Here's how the part is built. I have some questions about the finished solid (model axes, mm). A direction names the side the tool comes from. Coordinates: 2 decimals unless noted, no trailing zeros. Write each loop counter-clockwise with the first axis right and the second up, starting at its lowest first coordinate (ties: lowest second). Pieces come first, ordered by that corner, then holes.
Item 1: Please list where these lines run through material, in increasing order: line 1 (X direction, y = 0.5, z = 3); line 2 (Z direction, x = 6.25, y = -1.5); line 3 (X direction, y = 2, z = -0.75).
Item 2: I'm going to push flat-ended pins straight in: P1, Ø1, axis at y = 2.5, z = 1.5, coming from the +X side; P2, Ø1, axis at x = 2.5, y = -1, coming from the +Z side; P3, Ø1.5, axis at x = 3.5, y = 2, coming from the +Z side. Where does each tip first touch, or does it pass through?
Item 3: I want a section at C-C (x = 5.75). Please give me the cut outline in (y, z).
Item 4: I want a section at A-A (z = 0). Please give me the cut outline in (x, y).
Item 5: If we mould it in two halves opening along X, with no side actions, what happens to faces 1 (the face through (4, 2, 0)), 2 (the face through (7, 0, 0)), 3 (the face through (1, 2, 2)), 4 (the face through (6.3, -0.1, -2.5))? For each: pulls with the +X half, pulls with the -X half, needs draft (parallel to the pull), parting line crosses it, or undercut.
Item 6: For faces 5 (the face through (6, -2, 1)), 6 (the face through (0, 0, 0)), which set-ups out of +Z, -Z, +X, -X, +Y, -Y let a thin tool reach every point of the face, with its end or its side?
from build123d import *

# Parameters (mm, degrees)
SMUSSO1_SIZE = 0.5


with BuildPart() as part:
    # Schizzo1 → Rivoluzione1 (revolve)
    with BuildSketch(Plane.XY, mode=Mode.PRIVATE) as rivoluzione1_sk:
        Polygon((0, 0), (0, 3.75), (1, 3.75), (1, 2), (6, 2), (6, 2.5), (7, 2.5), (7, 0), align=None)
    revolve(rivoluzione1_sk.sketch.rotate(Axis((-5.173483989, 0, 0), (1, 0, 0)), 90), axis=Axis((-5.173483989, 0, 0), (1, 0, 0)))

    # Smusso1
    smusso1_edges = [part.edges().sort_by_distance(p)[0] for p in [
        (7, 0, -2.5),
        (0, 0, -3.75),
    ]]
    chamfer(smusso1_edges, length=SMUSSO1_SIZE)


solid = part.part
Answer:
1. line 1: x = 0 to 1
1. line 2: z = -2 to 2
1. line 3: x = 0 to 1, 6 to 6.86
2. P1: stops at x = 6.58
2. P2: stops at z = 1.94
2. P3: stops at z = 1.56
3. outline: circle Ø4 at (0, 0)
4. outline: (0, -3.25) - (0.5, -3.75) - (1, -3.75) - (1, -2) - (6, -2) - (6, -2.5) - (6.5, -2.5) - (7, -2) - (7, 2) - (6.5, 2.5) - (6, 2.5) - (6, 2) - (1, 2) - (1, 3.75) - (0.5, 3.75) - (0, 3.25) - close
5. face 1: undercut
5. face 2: pulls with the +X half
5. face 3: undercut
5. face 4: needs draft
6. face 5: none
6. face 6: +Z, -Z, -X, +Y, -Y
